CAD build for the part. Positions are in the model's coordinates, mm. A direction names the side the tool comes from. Coordinates: 2 decimals unless noted, no trailing zeros. Loops run counter-clockwise (first coordinate to the right, second up) from the corner with the lowest first, then second, coordinate; pieces in that order, holes last.
1) Saw through at A-A, the plane z = 20. Write the cut outline in (x, y) (3 decimals).
2) Saw through at B-B, the plane x = -8.15. Write the cut outline in (y, z), and give its area (3 significant figures).
3) Which spindle directions (+Z, -Z, +X, -X, +Y, -Y) get a long thin tool onto all of the face, cutting with end or side? Do faces 4 (the flat face through (16.15, 0, 9)), 5 (the flat face through (-16.15, 0, 9)), 6 (the flat face through (-16.15, 0, 24)), 7 (the flat face through (0, 7.65, 14)), 8 (the flat face through (16.15, 0, 24)). Say none if no direction does.
4) Saw through at D-D, the plane x = 18.5. Write the cut outline in (y, z).
5) Pin check, flat tips, straight feed: pin 1 Ø12 at (x, y) = (11.5, 11) entering from -Z; pin 2 Ø1.5 at (y, z) = (2.5, 11.5) entering from -X; pin 3 Ø5 at (x, y) = (19.375, 3.75) entering from -Z; pin 4 Ø3.5 at (y, z) = (2.5, 25) entering from +X. Stop position of each tip, or through.
6) Wall check: line 1 along Y through (x, z) = (12, 22); line 2 along Z through (x, y) = (-19.5, 0.5); line 3 along Z through (x, y) = (14.5, -1). Give the ranges that are in metal, low to high.
7) Saw through at C-C, the plane y = 13. Write the cut outline in (x, z).
8) Two-plate mould, pull along X, no slides. Class faces 1 (the cylindrical face through (-3.524, 1.457, 29.818)), 2 (the flat face through (-8, 11, 32.1)), 3 (the cylindrical face through (17.427, -3.664, 19.986)): +X half, -X half, draft (parallel to the pull), parting line (faces both ways), or undercut.
```python
from build123d import *

# Parameters (mm, degrees)
F0_W     = 32.3
F0_H     = 15.3
F1_DEPTH = 27.6
F3_W     = 44
F3_H     = 15.3
F3_R     = 1.95
F4_DEPTH = 2
F5_R     = 4.85
F6_DEPTH = 4.5
F7_R     = 1.25
F8_DEPTH = 2.5


with BuildPart() as f1:
    # F0 (on Top) → F1 (new body)
    with BuildSketch(Plane.XY):
        Rectangle(F0_W, F0_H)
    extrude(amount=F1_DEPTH)

    # F3 (on offset) → F4 (join)
    with BuildSketch(Plane.XY.offset(19)):
        Rectangle(F3_W, F3_H)
        with Locations((-19.375, -3.75)):
            Circle(F3_R, mode=Mode.SUBTRACT)
        with Locations((19.375, -3.75)):
            Circle(F3_R, mode=Mode.SUBTRACT)
        with Locations((-19.375, 3.75)):
            Circle(F3_R, mode=Mode.SUBTRACT)
        with Locations((19.375, 3.75)):
            Circle(F3_R, mode=Mode.SUBTRACT)
    extrude(amount=F4_DEPTH)

    # F5 (on face) → F6 (join)
    with BuildSketch(Plane.XY.offset(27.6)):
        with Locations((-8.15, 0)):
            Circle(F5_R)
    extrude(amount=F6_DEPTH)

    # F7 (on face) → F8 (join)
    with BuildSketch(Plane.XY.offset(32.1)):
        with BuildLine():
            ThreePointArc((-14.00677, 0.712917), (-8.507113, -5.889182), (-2.25, 0))
            ThreePointArc((-2.25, 0), (-2.260818, 0.357113), (-2.29323, 0.712917))
            ThreePointArc((-2.29323, 0.712917), (-8.15, 5.9), (-14.00677, 0.712917))
        make_face()
        with BuildLine():
            ThreePointArc((-14.00677, 0.712917), (-8.15, 5.9), (-2.29323, 0.712917))
            Line((-2.29323, 0.712917), (-5.171982, 24.3625))
            ThreePointArc((-5.171982, 24.3625), (-5.1555, 24.181583), (-5.15, 24))
            ThreePointArc((-5.15, 24), (-8.331583, 21.0055), (-11.128018, 24.3625))
            Line((-11.128018, 24.3625), (-14.00677, 0.712917))
        make_face()
        with Locations((-8.15, 13)):
            Circle(F7_R, mode=Mode.SUBTRACT)
        with BuildLine():
            ThreePointArc((-5.15, 24), (-5.1555, 24.181583), (-5.171982, 24.3625))
            ThreePointArc((-5.171982, 24.3625), (-8.15, 27), (-11.128018, 24.3625))
            ThreePointArc((-11.128018, 24.3625), (-8.331583, 21.0055), (-5.15, 24))
        make_face()
    extrude(amount=F8_DEPTH)


solid = f1.part
```
Data:
1. outline: (-22, -7.65) - (22, -7.65) - (22, 7.65) - (-22, 7.65) - close; hole circle Ø3.9 at (-19.375, -3.75); hole circle Ø3.9 at (-19.375, 3.75); hole circle Ø3.9 at (19.375, -3.75); hole circle Ø3.9 at (19.375, 3.75)
2. outline: (-7.65, 0) - (7.65, 0) - (7.65, 27.6) - (4.85, 27.6) - (4.85, 32.1) - (11.75, 32.1) - (11.75, 34.6) - (-5.9, 34.6) - (-5.9, 32.1) - (-4.85, 32.1) - (-4.85, 27.6) - (-7.65, 27.6) - close; (14.25, 32.1) - (27, 32.1) - (27, 34.6) - (14.25, 34.6) - close
2. area: 542 mm2
3. face 4: -Z, +X, +Y, -Y
3. face 5: -Z, -X, +Y, -Y
3. face 6: +Z, -X, +Y, -Y
3. face 7: -Z, +X, -X, +Y
3. face 8: +Z, +X, +Y, -Y
4. outline: (-7.65, 19) - (-5.49, 19) - (-5.49, 21) - (-7.65, 21) - close; (-2.01, 19) - (2.01, 19) - (2.01, 21) - (-2.01, 21) - close; (5.49, 19) - (7.65, 19) - (7.65, 21) - (5.49, 21) - close
5. pin 1: stops at z = 0
5. pin 2: stops at x = -16.15
5. pin 3: stops at z = 19
5. pin 4: stops at x = 16.15
6. line 1: y = -7.65 to 7.65
6. line 2: z = 19 to 21
6. line 3: z = 0 to 27.6
7. outline: (-12.51, 32.1) - (-9.4, 32.1) - (-9.4, 34.6) - (-12.51, 34.6) - close; (-6.9, 32.1) - (-3.79, 32.1) - (-3.79, 34.6) - (-6.9, 34.6) - close
8. face 1: parting line
8. face 2: draft
8. face 3: undercut
